```python
from build123d import *

# Parameters (mm, degrees)
F0_R     = 50.8
F1_DEPTH = 50.8
F2_R     = 25.4
F3_DEPTH = 101.601
F6_R     = 5.08
F7_R     = 5.08


with BuildPart() as f1:
    # F0 (on Right) → F1 (new body, symmetric)
    with BuildSketch(Plane.YZ):
        Circle(F0_R)
    extrude(amount=F1_DEPTH, both=True)

    # F2 (on face) → F3 (cut, through all)
    with BuildSketch(Plane.YZ.offset(50.8)):
        Circle(F2_R)
    extrude(amount=-F3_DEPTH, mode=Mode.SUBTRACT)

    # F4 (on Front) → F5 (revolve, cut)
    with BuildSketch(Plane.XZ):
        Polygon((38.1, 50.8), (-38.1, 50.8), (0, 31.75), align=None)
    revolve(axis=Axis((-4.27404, 0, 0), (1, 0, 0)), mode=Mode.SUBTRACT)

    # F6
    f6_edges = [f1.edges().sort_by_distance(p)[0] for p in [
        (0, 0, -31.75),
    ]]
    fillet(f6_edges, radius=F6_R)

    # F7
    f7_edges = [f1.edges().sort_by_distance(p)[0] for p in [
        (38.1, -35.921024, -35.921024),
        (50.8, -50.8, 0),
        (-38.1, -35.921024, -35.921024),
        (-50.8, -50.8, 0),
    ]]
    fillet(f7_edges, radius=F7_R)


solid = f1.part
```
Could you check a few things on this model? Use its own coordinates, in mm. A direction names the side the tool comes from. Round coordinates to 2 decimals unless told otherwise and drop trailing zeros. Loops run counter-clockwise (first coordinate to the right, second up) from the corner with the lowest first, then second, coordinate; pieces in that order, holes last. Notation, with made-up numbers: M 12.5,77.5 L 48.5,77.5 A3 ccw 48.5,81.5 Z; hole C 3.5,31.5 d2. An arc over 180 degrees is marked long. Put each result on its own line as item: value.
Q1. Imagine slicing it at B-B (x = 16). Write out the boundary of the cut face in (y, z).
Check result:
outline: C 0,0 d79.5; hole C 0,0 d50.8
Q2. Imagine slicing it at A-A (x = -29.5). Write out the boundary of the cut face in (y, z).
Check result:
outline: C 0,0 d93; hole C 0,0 d50.8
Q3. On a 3-axis mill with a long thin cutter (end or side, diameter ignored), from which of +Z, -Z, +X, -X, +Y, -Y can I reach the whole of each face in a straight line? I mean faces 4 (the face through (-42.464, 46.926, -19.457)), 5 (the face through (4.446, 13.012, 31.382)). Say none if no direction works.
Check result:
face 4: +X, -X
face 5: none
Q4. For pin 1 (1 mm diameter, centred on x = -34.5, z = 39, fed in from +Y); pin 2 (5 mm diameter, centred on x = 13, y = -3, fed in from +Z); pin 3 (10 mm diameter, centred on x = 21.5, y = 11.5, fed in from +Z), each with a flat end and sliding along its axis, tell me the tip position at first contact or that it passes through.
Check result:
pin 1: y = 30.43
pin 2: z = 39.4
pin 3: z = 43.77
Q5. I need wall thicknesses on probe 1 along X at (y, z) = (-43, -9); probe 2 along X at (y, z) = (-25, 28.5); probe 3 along Y at (x, z) = (-24.5, 21). Which ranges of each line are inside material? Lowest first, please.
Check result:
probe 1: -50.8 to -24.36, 24.36 to 50.8
probe 2: -50.8 to -12.32, 12.32 to 50.8
probe 3: -38.67 to -14.29, 14.29 to 38.67
Q6. Thinking about a two-plate mould opening in Z: for faces 1 (the face through (0.711, -5.506, -24.796)), 2 (the face through (42.554, 46.926, -19.457)), 3 (the face through (50.8, 20, -20)), which applies, released by +Z, released by -Z, zero draft, split by the parting line, or undercut?
Check result:
face 1: undercut
face 2: split by the parting line
face 3: zero draft
